Design review of the part built by this model. Coordinates are the model's own, in mm. Face numbers are marked on the shaded views. A direction names the side the tool comes from. Give positions to 0.01 mm unless a question says otherwise; leave off trailing zeros. Order: outer loops, then holes, each group sorted by start corner. A loop starts at its lowest first (then second) coordinate and runs counter-clockwise, first axis right, second up.
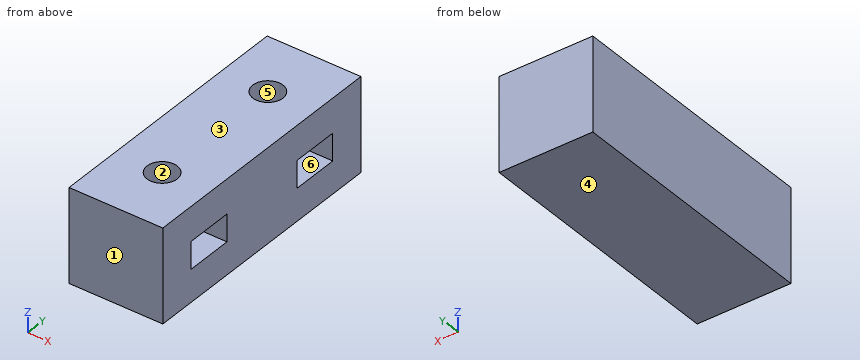
```python
from build123d import *

# Parameters (mm, degrees)
SKETCH1_W           = 25.4
SKETCH1_H           = 25.4
SKETCH1_W_2         = 12.7
SKETCH1_H_2         = 6.858
BOSS_EXTRUDE1_DEPTH = 71.374
SKETCH2_R           = 4.09575
CUT_EXTRUDE1_DEPTH  = 19.05
SKETCH5_W           = 7.366
SKETCH5_H           = 12.954
CUT_EXTRUDE2_DEPTH  = 19.05


with BuildPart() as part:
    # Sketch1 → Boss-Extrude1 (new body)
    # profile 1 of 2: a face of its own
    with BuildSketch(Plane(origin=(0, 0, 0), x_dir=(1, 0, 0), z_dir=(0, 1, 0))):
        with Locations((12.7, 12.7)):
            Rectangle(SKETCH1_W, SKETCH1_H)
        with Locations((12.7, 12.7)):
            Rectangle(SKETCH1_W_2, SKETCH1_H_2, mode=Mode.SUBTRACT)
    # profile 2 of 2: a face of its own
    with BuildSketch(Plane(origin=(0, 0, 0), x_dir=(1, 0, 0), z_dir=(0, 1, 0))):
        with Locations((12.7, 12.7)):
            Rectangle(SKETCH1_W_2, SKETCH1_H_2)
    extrude(amount=BOSS_EXTRUDE1_DEPTH)

    # Sketch2 → Cut-Extrude1 (cut)
    with BuildSketch(Plane.XY):
        with Locations((12.7, 54.737)):
            Circle(SKETCH2_R)
        with Locations((12.7, 16.637)):
            Circle(SKETCH2_R)
    extrude(amount=-CUT_EXTRUDE1_DEPTH, mode=Mode.SUBTRACT)

    # Sketch5 → Cut-Extrude2 (cut)
    with BuildSketch(Plane(origin=(25.4, 0, 0), x_dir=(0, 0, -1), z_dir=(1, 0, 0))):
        with Locations((12.954, 54.737)):
            Rectangle(SKETCH5_W, SKETCH5_H)
        with Locations((12.954, 16.637)):
            Rectangle(SKETCH5_W, SKETCH5_H)
    extrude(amount=-CUT_EXTRUDE2_DEPTH, mode=Mode.SUBTRACT)


solid = part.part
```
1. Take a section at D-D (x = 12.7). State the section outline as (y, z) points.
Recorded:
outline: (0, -25.4) - (71.37, -25.4) - (71.37, 0) - (58.83, 0) - (58.83, -9.27) - (61.21, -9.27) - (61.21, -16.64) - (58.83, -16.64) - (58.83, -19.05) - (50.64, -19.05) - (50.64, -16.64) - (48.26, -16.64) - (48.26, -9.27) - (50.64, -9.27) - (50.64, 0) - (20.73, 0) - (20.73, -9.27) - (23.11, -9.27) - (23.11, -16.64) - (20.73, -16.64) - (20.73, -19.05) - (12.54, -19.05) - (12.54, -16.64) - (10.16, -16.64) - (10.16, -9.27) - (12.54, -9.27) - (12.54, 0) - (0, 0) - close
2. For line 1 along Y through (x, z) = (12.7, -2.75); line 2 along Y through (x, z) = (19.5, -9.5), list the stretches that pass through material, from the lowest coordinate up.
Recorded:
line 1: y = 0 to 12.54, 20.73 to 50.64, 58.83 to 71.37
line 2: y = 0 to 10.16, 23.11 to 48.26, 61.21 to 71.37
3. Take a section at B-B (z = -11.5). State the section outline as (x, y) points, then the cut area to 3 significant figures.
Recorded:
outline: (0, 0) - (25.4, 0) - (25.4, 10.16) - (6.35, 10.16) - (6.35, 23.11) - (25.4, 23.11) - (25.4, 48.26) - (6.35, 48.26) - (6.35, 61.21) - (25.4, 61.21) - (25.4, 71.37) - (0, 71.37) - close
area: 1,320 mm2
4. Machinability: for the marked faces 4, 5 and 6, which of the approach directions +Z, -Z, +X, -X, +Y, -Y give a long, thin tool a straight path to every point of the face, cutting with its end or side? Answer none if there is none.
Recorded:
face 4: -Z, +X, -X, +Y, -Y
face 5: +Z
face 6: +X
5. For pin 1 (12 mm diameter, centred on x = 18.5, z = -20.5, fed in from -Y); pin 2 (2.5 mm diameter, centred on x = 14.5, y = 54, fed in from +Z); pin 3 (2 mm diameter, centred on y = 52.5, z = -12, fed in from +X), all flat-tipped, find the tip position at first contact; note any pin that passes through.
Recorded:
pin 1: stops at y = 0
pin 2: stops at z = -19.05
pin 3: stops at x = 6.35
6. Take a section at C-C (y = 11.5). State the section outline as (x, z) points.
Recorded:
outline: (0, -25.4) - (25.4, -25.4) - (25.4, -16.64) - (6.35, -16.64) - (6.35, -9.27) - (25.4, -9.27) - (25.4, 0) - (0, 0) - close
7. Take a section at A-A (x = 18). State the section outline as (y, z) points, then the cut area to 3 significant figures.
Recorded:
outline: (0, -25.4) - (71.37, -25.4) - (71.37, 0) - (0, 0) - close; hole (10.16, -16.64) - (23.11, -16.64) - (23.11, -9.27) - (10.16, -9.27) - close; hole (48.26, -16.64) - (61.21, -16.64) - (61.21, -9.27) - (48.26, -9.27) - close
area: 1,620 mm2
8. Draft analysis for pull direction Y (two halves, no side actions). For the marked faces 1, 2 and 3, state which applies: pulls with the +Y half, pulls with the -Y half, needs draft (parallel to the pull), parting line crosses it, or undercut.
Recorded:
face 1: pulls with the -Y half
face 2: undercut
face 3: needs draft
